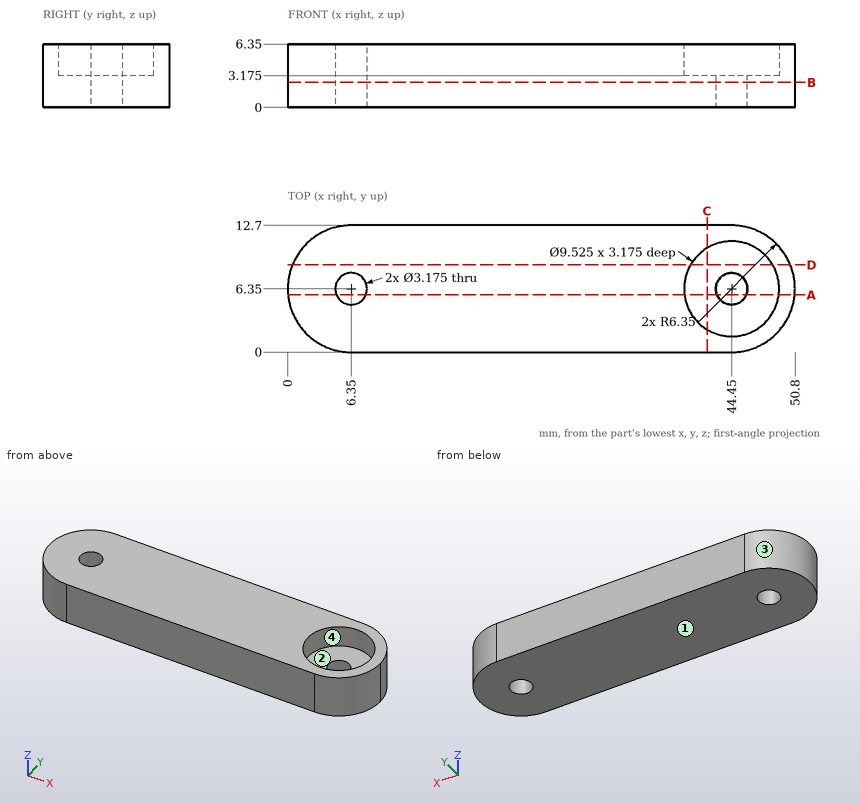
Geometry check sheet. Reference: drawing and pictorial views, mm from the part's lowest x, y, z. Round coordinates to 2 decimals unless told otherwise and drop trailing zeros. Loops run counter-clockwise (first coordinate to the right, second up) from the corner with the lowest first, then second, coordinate; pieces in that order, holes last. Notation, with made-up numbers: (1, -34.75) -> (60, -34.75) arc R31 ccw to (60, -2.75) -> close; hole circle Ø8 at (34, 12). An arc over 180 degrees is marked (long way). Use a Markdown table: item, result.
(1) Sectioned sample at C-C (x = 42). Enter the section's corners in (y, z) (3 decimals), then the cut area to 3 significant figures.
Calculated:
| item | result |
|---|---|
| outline | (0, 0) -> (12.7, 0) -> (12.7, 6.35) -> (10.434, 6.35) -> (10.434, 3.175) -> (2.266, 3.175) -> (2.266, 6.35) -> (0, 6.35) -> close |
| area | 54.7 mm² |
(2) Mould release check, pull along X, two halves, no side actions. Record for the marked faces 1, 2, 3 and 4: released by +X, released by -X, zero draft, split by the parting line, or undercut.
Calculated:
| item | result |
|---|---|
| face 1 | zero draft |
| face 2 | undercut |
| face 3 | released by -X |
| face 4 | undercut |
(3) Sectioned sample at B-B (z = 2.5). Give the number of separate pieces and of enclosed holes in the cut face, then the cut area to 3 significant figures.
Calculated:
| item | result |
|---|---|
| separate pieces | 1 |
| enclosed holes | 2 |
| area | 595 mm² |
(4) Scan lines: probe 1 along Y at (x, z) = (44.45, 1.55); probe 2 along X at (y, z) = (5.25, 2.5); probe 3 along Y at (x, z) = (42.5, 5). Record each from-to range of solid material in increasing order.
Calculated:
| item | result |
|---|---|
| probe 1 | 0 to 4.76, 7.94 to 12.7 |
| probe 2 | 0.1 to 5.21, 7.49 to 43.31, 45.59 to 50.7 |
| probe 3 | 0 to 2.01, 10.69 to 12.7 |
(5) Sectioned sample at A-A (y = 5.75). Enter the section's corners in (x, z) (3 decimals), then the cut area to 3 significant figures.
Calculated:
| item | result |
|---|---|
| outline | (0.028, 0) -> (4.88, 0) -> (4.88, 6.35) -> (0.028, 6.35) -> close; (7.82, 0) -> (42.98, 0) -> (42.98, 3.175) -> (39.725, 3.175) -> (39.725, 6.35) -> (7.82, 6.35) -> close; (45.92, 0) -> (50.772, 0) -> (50.772, 6.35) -> (49.175, 6.35) -> (49.175, 3.175) -> (45.92, 3.175) -> close |
| area | 264 mm² |
(6) Go/stop test with flat-tipped pins: P1, Ø2, axis at y = 9.5, z = 1.5, coming from the +X side; P2, Ø7.5, axis at x = 44.45, y = 6.35, coming from the +Z side (3 decimals); P3, Ø2, axis at y = 3, z = 1.5, coming from the +X side. Record where each tip stops, or that it passes through.
Calculated:
| item | result |
|---|---|
| P1 | x = 50.42 |
| P2 | z = 3.175 |
| P3 | x = 50.35 |
(7) Sectioned sample at D-D (y = 8.75). Enter the section's corners in (x, z) (3 decimals).
Calculated:
| item | result |
|---|---|
| outline | (0.471, 0) -> (50.329, 0) -> (50.329, 6.35) -> (48.564, 6.35) -> (48.564, 3.175) -> (40.336, 3.175) -> (40.336, 6.35) -> (0.471, 6.35) -> close |
